Check sheet for the modelled part. Datum: model origin and axes. Units: mm. Face numbers are marked on the shaded views. Give positions to 0.01 mm unless a question says otherwise; leave off trailing zeros. Order: outer loops, then holes, each group sorted by start corner. A loop starts at its lowest first (then second) coordinate and runs counter-clockwise, first axis right, second up. Notation, with made-up numbers: (-33.5, 21) - (3.5, 21) arc R26 cw to (3.5, 59) - close; hole circle Ø3 at (24.5, 79.5). An arc over 180 degrees is marked (long way). Answer in a Markdown table with one row per item.
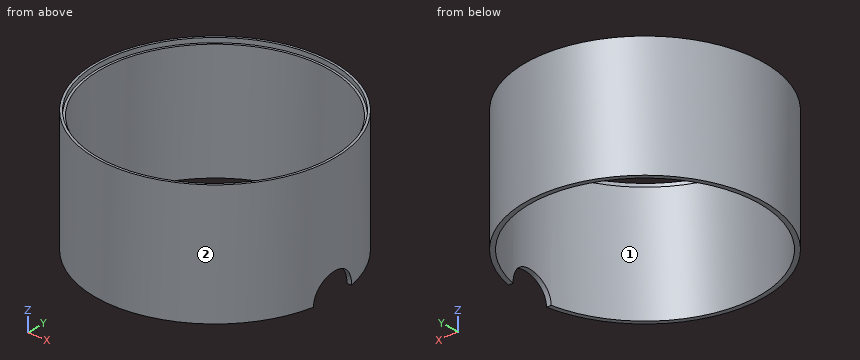
from build123d import *

# Parameters (mm, degrees)
CYLINDER009_R           = 51
CYLINDER009_DEPTH       = 16
CYLINDER006_R           = 10
CYLINDER006_DEPTH       = 10
CYLINDER006_PITCH_ANGLE = 90
CYLINDER005_R           = 50
CYLINDER005_DEPTH       = 67
CYLINDER004_R           = 52
CYLINDER004_DEPTH       = 53


with BuildPart() as cylinder004:
    # Cylinder009 → Cylinder009 (new body)
    with BuildSketch(Plane.XY.offset(51)):
        Circle(CYLINDER009_R)
    extrude(amount=CYLINDER009_DEPTH)


with BuildPart() as wire_hole:
    # Cylinder006 → Cylinder006 (new body)
    with BuildSketch(Plane.XY):
        Circle(CYLINDER006_R)
    extrude(amount=CYLINDER006_DEPTH)


with BuildPart() as wire_hole_1:
    # Cylinder006 pitch: moved
    add(wire_hole.part.rotate(Axis((0, 0, 0), (0, 1, 0)), CYLINDER006_PITCH_ANGLE))


with BuildPart() as wire_hole_2:
    # Cylinder006 placement: moved
    add(wire_hole_1.part.moved(Location((45, 0, 0))))


with BuildPart() as inner:
    # Cylinder005 → Cylinder005 (new body)
    with BuildSketch(Plane.XY):
        Circle(CYLINDER005_R)
    extrude(amount=CYLINDER005_DEPTH)


with BuildPart() as case_with_edge:
    # Cylinder004 → Cylinder004 (new body)
    with BuildSketch(Plane.XY):
        Circle(CYLINDER004_R)
    extrude(amount=CYLINDER004_DEPTH)

    # Cut002: cut Inner
    add(inner.part, mode=Mode.SUBTRACT)

    # Cut003: cut Wire hole
    add(wire_hole_2.part, mode=Mode.SUBTRACT)

    # Cut005: cut Cylinder004
    add(cylinder004.part, mode=Mode.SUBTRACT)


solid = case_with_edge.part
(1) Cross-section at B-B, the plane x = 0. Record the cut outline in (y, z), then the cut area to 3 significant figures.
Geometry says:
| item | result |
|---|---|
| outline | (-52, 0) - (-50, 0) - (-50, 51) - (-51, 51) - (-51, 53) - (-52, 53) - close; (50, 0) - (52, 0) - (52, 53) - (51, 53) - (51, 51) - (50, 51) - close |
| area | 208 mm² |
(2) Gauge pin test, flat ends, axial feed: P1, Ø4, axis at x = 14, z = 21, coming from the +Y side; P2, Ø4, axis at x = -38, z = 9, coming from the +Y side; P3, Ø1, axis at x = 4, z = 44.5, coming from the +Y side. Record the tip position at first contact, or that the pin passes through.
Geometry says:
| item | result |
|---|---|
| P1 | y = 50.6 |
| P2 | y = 37.52 |
| P3 | y = 51.88 |
(3) Thickness scan on L1, parallel to Y at x = 0, z = 39.5; L2, parallel to X at y = 0, z = 52. Record the ranges inside material, lowest first.
Geometry says:
| item | result |
|---|---|
| L1 | -52 to -50, 50 to 52 |
| L2 | -52 to -51, 51 to 52 |
(4) Mould release check, pull along X, two halves, no side actions. Record for the marked faces 1 and 2: pulls with the +X half, pulls with the -X half, needs draft (parallel to the pull), parting line crosses it, or undercut.
Geometry says:
| item | result |
|---|---|
| face 1 | undercut |
| face 2 | parting line crosses it |
(5) Cross-section at A-A, the plane y = 0. Record the cut outline in (x, z).
Geometry says:
| item | result |
|---|---|
| outline | (-52, 0) - (-50, 0) - (-50, 51) - (-51, 51) - (-51, 53) - (-52, 53) - close; (50, 10) - (52, 10) - (52, 53) - (51, 53) - (51, 51) - (50, 51) - close |
(6) Cross-section at C-C, the plane z = 22. Record the cut outline in (x, y), then the cut area to 3 significant figures.
Geometry says:
| item | result |
|---|---|
| outline | circle Ø104 at (0, 0); hole circle Ø100 at (0, 0) |
| area | 641 mm² |
